```python
from build123d import *

# Parameters (mm, degrees)
F0_W     = 203.2
F0_H     = 50.8
F1_DEPTH = 127
F2_W     = 50.8
F2_H     = 76.2
F3_DEPTH = 101.6
F4_W     = 50.8
F4_H     = 76.2
F5_DEPTH = 101.6
F6_W     = 101.6
F6_H     = 50.8
F7_DEPTH = 25.4
F8_W     = 101.6
F8_H     = 25.4
F9_DEPTH = 101.6


with BuildPart() as f1:
    # F0 (on Front) → F1 (new body)
    with BuildSketch(Plane.XZ):
        with Locations((0.721672, -31.288108)):
            Rectangle(F0_W, F0_H)
    extrude(amount=F1_DEPTH)

    # F2 (on face) → F3 (join)
    with BuildSketch(Plane.XY.offset(-5.888108)):
        with Locations((-75.478328, -38.1)):
            Rectangle(F2_W, F2_H)
    extrude(amount=F3_DEPTH)

    # F4 (on face) → F5 (join)
    with BuildSketch(Plane.XY.offset(-5.888108)):
        with Locations((76.921672, -38.1)):
            Rectangle(F4_W, F4_H)
    extrude(amount=F5_DEPTH)

    # F6 (on face) → F7 (join)
    with BuildSketch(Plane.XY.offset(-5.888108)):
        with Locations((0.721672, -50.8)):
            Rectangle(F6_W, F6_H)
    extrude(amount=F7_DEPTH)

    # F8 (on face) → F9 (join)
    with BuildSketch(Plane.XY.offset(-5.888108)):
        with Locations((0.721672, -12.7)):
            Rectangle(F8_W, F8_H)
    extrude(amount=F9_DEPTH)


solid = f1.part
```
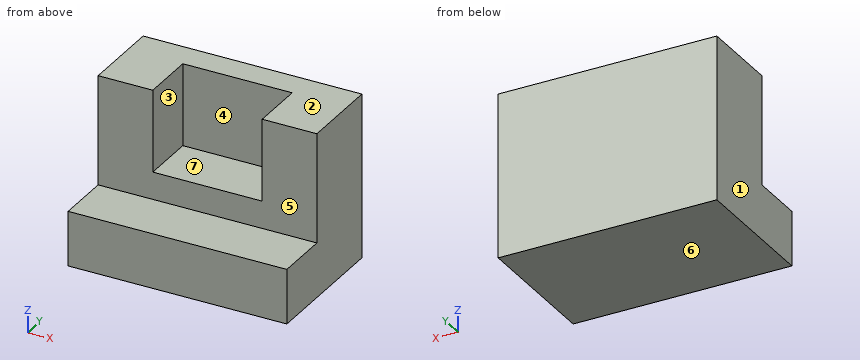
Design review of the part built by this model. Coordinates are the model's own, in mm. Face numbers are marked on the shaded views. A direction names the side the tool comes from. Coordinates: 2 decimals unless noted, no trailing zeros. Loops run counter-clockwise (first coordinate to the right, second up) from the corner with the lowest first, then second, coordinate; pieces in that order, holes last. Notation, with made-up numbers: M 10,42 L 59,42 A15 cw 59,71 Z; hole C 58,-20.75 d6. An arc over 180 degrees is marked long. One line per question, with ' | ' between items.
(1) We need section D-D (x = 56). Give the boundary of the cut face in (y, z), and give its area (3 significant figures).
Filled in:
outline: M -127,-56.69 L 0,-56.69 L 0,95.71 L -76.2,95.71 L -76.2,-5.89 L -127,-5.89 Z | area: 14,200 mm^2
(2) We need section A-A (x = 29). Give the boundary of the cut face in (y, z).
Filled in:
outline: M -127,-56.69 L 0,-56.69 L 0,95.71 L -25.4,95.71 L -25.4,19.51 L -76.2,19.51 L -76.2,-5.89 L -127,-5.89 Z
(3) Wall thickness on probe 1 along X at (y, z) = (-28, 20); probe 2 along Z at (x, y) = (-43, -38.5); probe 3 along Z at (x, y) = (-21.5, -97): over which ranges is each line inside the solid? List them lowest first.
Filled in:
probe 1: x = -100.88 to -50.08, 51.52 to 102.32 | probe 2: z = -56.69 to 19.51 | probe 3: z = -56.69 to -5.89
(4) We need section C-C (z = 7.5). Give the boundary of the cut face in (x, y), and give its area (3 significant figures).
Filled in:
outline: M -100.88,-76.2 L 102.32,-76.2 L 102.32,0 L -100.88,0 Z | area: 15,500 mm^2
(5) We need section B-B (y = -29). Give the boundary of the cut face in (x, z).
Filled in:
outline: M -100.88,-56.69 L 102.32,-56.69 L 102.32,95.71 L 51.52,95.71 L 51.52,19.51 L -50.08,19.51 L -50.08,95.71 L -100.88,95.71 Z
(6) Draft analysis for pull direction X (two halves, no side actions). For the marked faces 1, 2, 3 and 4, state which applies: released by +X, released by -X, zero draft, split by the parting line, or undercut.
Filled in:
face 1: released by -X | face 2: zero draft | face 3: undercut | face 4: undercut
(7) For pin 1 Ø4 at (x, z) = (-62.5, 43) entering from -Y; pin 2 Ø8 at (x, y) = (-21.5, -29.5) entering from +Z; pin 3 Ø23 at (x, z) = (-21, 56) entering from -Y, all flat-tipped, find the tip position at first contact; note any pin that passes through.
Filled in:
pin 1: stops at y = -76.2 | pin 2: stops at z = 19.51 | pin 3: stops at y = -25.4
(8) Machinability: for the marked faces 5, 6 and 7, which of the approach directions +Z, -Z, +X, -X, +Y, -Y give a long, thin tool a straight path to every point of the face, cutting with its end or side? Answer none if there is none.
Filled in:
face 5: +Z, +X, -X, -Y | face 6: -Z, +X, -X, +Y, -Y | face 7: +Z, -Y
